Autodesk Inventor part; units mm, degrees
ref_plane "YZ Plane" through (0, 0, 0) normal (1, 0, 0) x (0, 1, 0)
ref_plane "XZ Plane" through (0, 0, 0) normal (0, 1, 0) x (-1, 0, 0)
ref_plane "XY Plane" through (0, 0, 0) normal (0, 0, 1) x (1, 0, 0)
sketch "Sketch1" plane through (0, 0, 0) normal (0, 1, 0) x (-1, 0, 0)
  circle A0 centre (0, 0) radius 38.5
  circle A1 centre (0, 0) radius 39.5
  dimension "d0" = 77
  dimension "d1" = 79
extrude "Extrusion1" add sketch "Sketch1" along normal blind 3
sketch "Sketch21" plane through (0, 3, 0) normal (0, 1, 0) x (1, 0, 0)
  line L0 (-39.5, -39.5) -> (39.5, -39.5)
  line L1 (39.5, -39.5) -> (39.5, 39.5)
  line L2 (39.5, 39.5) -> (-39.5, 39.5)
  line L3 (-39.5, 39.5) -> (-39.5, -39.5)
  line L4 (-39.5, -39.5) -> (39.5, 39.5) construction
  line L5 (39.5, -39.5) -> (-39.5, 39.5) construction
  circle A0 centre (0, 0) radius 39.5
  dimension "d111" = 79
  dimension "d112" = 79
extrude "Extrusion21" add sketch "Sketch21" against normal blind 3 contours L3 A0 L0 | A0 L1 L0 | L3 L2 A0 | A0 L2 L1
fillet "Fillet3" radius 20 4 edges at (-39.5, 1.5, -39.5) (39.5, 1.5, -39.5) (39.5, 1.5, 39.5) (-39.5, 1.5, 39.5)
properties part number "Motor mount (plain)"
Geometry check sheet. Reference: the model listing, model coordinates, mm. Give positions to 0.01 mm unless a question says otherwise; leave off trailing zeros. Loops run counter-clockwise (first coordinate to the right, second up) from the corner with the lowest first, then second, coordinate; pieces in that order, holes last. Notation, with made-up numbers: (18, 30.5) -> (72, 30.5) arc R23 cw to (72, 46.5) -> close; hole circle Ø11 at (27.25, 8). An arc over 180 degrees is marked (long way). Answer in a Markdown table with one row per item. Add a question column.
1) Cross-section at A-A on x = 0. Record the boundary of the cut face in (y, z).
2) Draft check along X on faces 1 (the face through (30.55, 1.48, 23.43)), 2 (the face through (33.797, 1.479, 33.486)), 3 (the face through (-33.797, 1.479, -33.486)), 4 (the face through (9, 0, -38)). Enter one of: pulls with the +X half, pulls with the -X half, needs draft (parallel to the pull), parting line crosses it, or undercut.
3) Material ranges on probe 1 along Z at (x, y) = (0, 1.9); probe 2 along X at (y, z) = (2.4, -25.5); probe 3 along X at (y, z) = (0.8, -33), recorded low to high. Write a range as from..to.
4) Cross-section at B-B on z = 0. Record the boundary of the cut face in (x, y), and give its area (3 significant figures).
5) Cross-section at C-C on y = 2.1. Record the boundary of the cut face in (x, z).
Outcome:
| question | item | result |
|---|---|---|
| 1 | outline | (0, -39.5) -> (3, -39.5) -> (3, -38.5) -> (0, -38.5) -> close; (0, 38.5) -> (3, 38.5) -> (3, 39.5) -> (0, 39.5) -> close |
| 2 | face 1 | undercut |
| 2 | face 2 | pulls with the +X half |
| 2 | face 3 | pulls with the -X half |
| 2 | face 4 | needs draft |
| 3 | probe 1 | z = -39.5..-38.5, 38.5..39.5 |
| 3 | probe 2 | x = -38.58..-28.84, 28.84..38.58 |
| 3 | probe 3 | x = -34.26..-19.83, 19.83..34.26 |
| 4 | outline | (-39.5, 0) -> (-38.5, 0) -> (-38.5, 3) -> (-39.5, 3) -> close; (38.5, 0) -> (39.5, 0) -> (39.5, 3) -> (38.5, 3) -> close |
| 4 | area | 6.00 mm^2 |
| 5 | outline | (-39.5, -19.5) arc R20 ccw to (-19.5, -39.5) -> (19.5, -39.5) arc R20 ccw to (39.5, -19.5) -> (39.5, 19.5) arc R20 ccw to (19.5, 39.5) -> (-19.5, 39.5) arc R20 ccw to (-39.5, 19.5) -> close; hole circle Ø77 at (0, 0) |
